Geometry check sheet. Reference: drawing and pictorial views, mm from the part's lowest x, y, z. Coordinates: 2 decimals unless noted, no trailing zeros. Order: outer loops, then holes, each group sorted by start corner. A loop starts at its lowest first (then second) coordinate and runs counter-clockwise, first axis right, second up. Notation, with made-up numbers: (-33.5, 86.5) -> (4.5, 86.5) arc R16 ccw to (4.5, 108.5) -> close; hole circle Ø11 at (-3, 30.5). An arc over 180 degrees is marked (long way). Use CSV: the item, a comma, the result in double quotes. Start each with the question number.
1) Sectioned sample at A-A on x = 152.4. Record the boundary of the cut face in (y, z).
2) Go/stop test with flat-tipped pins: pin 1 (13.5 mm diameter, centred on x = 12.7, y = 12.7, fed in from -Z); pin 2 (9.5 mm diameter, centred on x = 152.4, y = 12.7, fed in from +Z) (3 decimals). Record where each tip stops, or that it passes through.
3) Sectioned sample at B-B on y = 12.7. Record the boundary of the cut face in (x, z), then the cut area to 3 significant figures.
4) Sectioned sample at C-C on z = 1.75. Record the boundary of the cut face in (x, y), then the cut area to 3 significant figures.
5) Scan lines: line 1 along X through (y, z) = (12.25, 7.5); line 2 along Y through (x, z) = (12.7, 4.25); line 3 along X through (y, z) = (10, 3.75). Record each from-to range of solid material in increasing order.
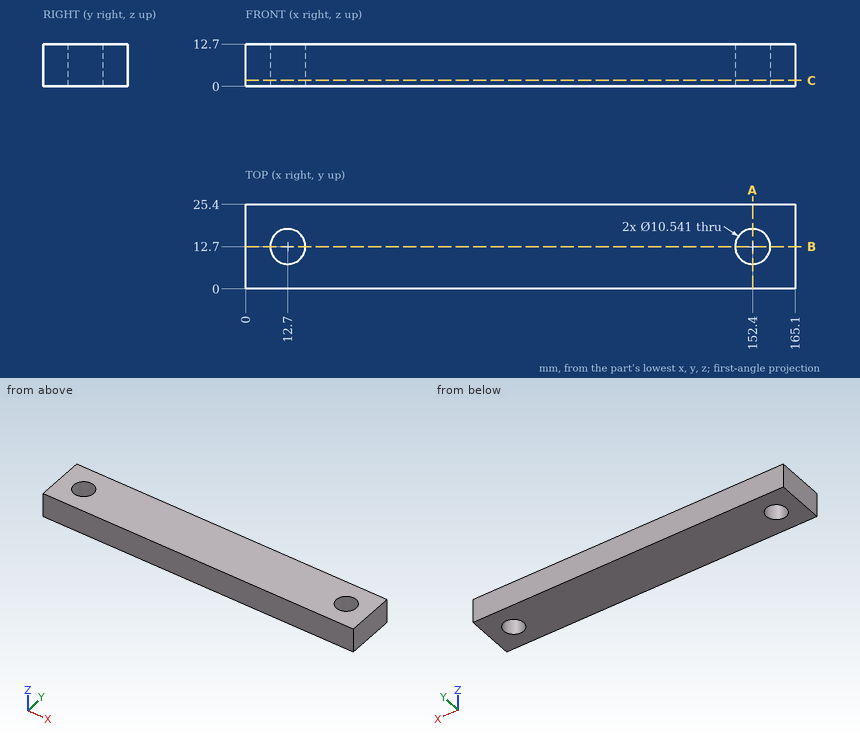
Answers follow:
1,outline,"(0, 0) -> (7.43, 0) -> (7.43, 12.7) -> (0, 12.7) -> close; (17.97, 0) -> (25.4, 0) -> (25.4, 12.7) -> (17.97, 12.7) -> close"
2,pin 1,"stops at z = 0"
2,pin 2,"passes through"
3,outline,"(0, 0) -> (7.43, 0) -> (7.43, 12.7) -> (0, 12.7) -> close; (17.97, 0) -> (147.13, 0) -> (147.13, 12.7) -> (17.97, 12.7) -> close; (157.67, 0) -> (165.1, 0) -> (165.1, 12.7) -> (157.67, 12.7) -> close"
3,area,"1,830 mm²"
4,outline,"(0, 0) -> (165.1, 0) -> (165.1, 25.4) -> (0, 25.4) -> close; hole circle Ø10.54 at (12.7, 12.7); hole circle Ø10.54 at (152.4, 12.7)"
4,area,"4,020 mm²"
5,line 1,"x = 0 to 7.45, 17.95 to 147.15, 157.65 to 165.1"
5,line 2,"y = 0 to 7.43, 17.97 to 25.4"
5,line 3,"x = 0 to 8.17, 17.23 to 147.87, 156.93 to 165.1"
